```python
from build123d import *
from build123d.topology import SkipClean

# Parameters (mm, degrees)
SKETCH1_W = 0.2413
SKETCH1_H = 2.286


with BuildPart() as part:
    # Sketch1 → Revolve1 (revolve)
    with SkipClean():  # the faces are left unmerged after this step: merging them gives an invalid solid
        with BuildSketch(Plane(origin=(0, 0, 0), x_dir=(1, 0, 0), z_dir=(0, 1, 0))):
            with BuildLine():
                ThreePointArc((0.7874, 0.7874), (0.55677588, 1.34417588), (0, 1.5748))
                Line((0, 1.5748), (0, 0))
                ThreePointArc((0, 0), (0.55677588, 0.23062412), (0.7874, 0.7874))
            make_face()
            with BuildLine():
                Line((0, 0), (0, 1.5748))
                ThreePointArc((0, 1.5748), (-0.7874, 0.7874), (0, 0))
            make_face()
            with BuildLine():
                Line((0.7874, 10.9728), (0, 10.9728))
                Line((0, 10.9728), (0, 1.5748))
                ThreePointArc((0, 1.5748), (0.55677588, 1.34417588), (0.7874, 0.7874))
                Line((0.7874, 0.7874), (0.7874, 10.9728))
            make_face()
            Polygon((0.7874, 11.6078), (0.5461, 11.6078), (0, 11.2903), (0, 10.9728), (0.7874, 10.9728), (1.4478, 10.9728), (1.4478, 11.6078), align=None)
            with Locations((0.66675, 12.7508)):
                Rectangle(SKETCH1_W, SKETCH1_H)
        revolve(axis=Axis((0, 0, 0), (0, 0, -1)))


solid = part.part
```
Check sheet for the modelled part. Datum: model origin and axes. Units: mm. A direction names the side the tool comes from. Give positions to 0.01 mm unless a question says otherwise; leave off trailing zeros. Write each loop counter-clockwise with the first axis right and the second up, starting at its lowest first coordinate (ties: lowest second). Pieces come first, ordered by that corner, then holes. Notation, with made-up numbers: (34, -23.5) - (83, -23.5) arc R24 cw to (83, -0.5) - close; hole circle Ø9 at (36.25, -33). An arc over 180 degrees is marked (long way). Answer as a JSON object with one key per item and string values. Group by question number.
1) Sectioned sample at B-B (z = -3). Record the cut outline in (x, y), then the cut area to 3 significant figures.
2) Sectioned sample at A-A (z = -12.5). Record the cut outline in (x, y), then the cut area to 3 significant figures.
3) Depth check by flat-ended pin: P1, Ø1.4, axis at x = 0, y = 0, coming from the -Z side. Enter the tip coordinate at first touch or a pass-through.
4) Sectioned sample at C-C (x = 0.95). Record the cut outline in (y, z), then the cut area to 3 significant figures.
5) Sectioned sample at D-D (x = -1.2). Record the cut outline in (y, z).
6) Thickness scan on probe 1 along X at (y, z) = (0, -13.1); probe 2 along Z at (x, y) = (-1.1, -0.35). Record the ranges inside material, lowest first. Write a range as from..to.
7) Access from +Z, -Z, +X, -X, +Y, -Y to the whole of each face (thin tool, end or side, straight path). Record for faces 1 (the face through (-0.314, 1.413, -11.295)), 2 (the face through (0, 1, -11.608)).
8) Release check for a two-part mould opening along X. For faces 3 (the face through (0, 1, -10.973)), 4 (the face through (-0.625, 0.479, -5.951)), 5 (the face through (-0.07, 0.05, -11.34)) record: pulls with the +X half, pulls with the -X half, needs draft (parallel to the pull), parting line crosses it, or undercut.
Geometry results:
{
 "1": {"outline": "circle Ø1.57 at (0, 0)", "area": "1.95 mm^2"},
 "2": {"outline": "circle Ø1.57 at (0, 0); hole circle Ø1.09 at (0, 0)", "area": "1.01 mm^2"},
 "3": {"P1": "stops at z = -13.89"},
 "4": {"outline": "(-1.09, -11.61) - (1.09, -11.61) - (1.09, -10.97) - (-1.09, -10.97) - close", "area": "1.39 mm^2"},
 "5": {"outline": "(-0.81, -11.61) - (0.81, -11.61) - (0.81, -10.97) - (-0.81, -10.97) - close"},
 "6": {"probe 1": "x = -0.79..-0.55, 0.55..0.79", "probe 2": "z = -11.61..-10.97"},
 "7": {"face 1": "+Z, -Z", "face 2": "-Z"},
 "8": {"face 3": "needs draft", "face 4": "parting line crosses it", "face 5": "undercut"}
}
